The listing builds one solid part. Answer for the finished solid, in the listing's coordinates (mm). Face numbers are marked on the shaded views. A direction names the side the tool comes from. Round coordinates to 2 decimals unless told otherwise and drop trailing zeros. Loops run counter-clockwise (first coordinate to the right, second up) from the corner with the lowest first, then second, coordinate; pieces in that order, holes last. Notation, with made-up numbers: (33.25, 70) - (59.25, 70) arc R24 cw to (59.25, 91) - close; hole circle Ø10 at (-17, -9.5). An arc over 180 degrees is marked (long way). Write item = value, one per line. Start each with the question number.
1) Section C-C, the plane z = -34 is taken. Determine the outline of the cut face in (x, y).
2) Section D-D, the plane x = 6.25 is taken. Determine the outline of the cut face in (y, z), and give its area (3 significant figures).
3) Straight lines are drawn through the part: line 1 along Z through (x, y) = (12, 5.25); line 2 along Y through (x, z) = (-3, -8); line 3 along Z through (x, y) = (-7, -5). For each, find the intervals that lie inside material, in ascending order.
4) Given pin 1 Ø1.5 at (x, y) = (0.5, -7) entering from -Z; pin 2 Ø12 at (x, z) = (8.5, -1.5) entering from +Y; pin 3 Ø1.5 at (x, z) = (6.5, -31.5) entering from -Y; pin 4 Ø2 at (x, y) = (-7, 1) entering from +Z, each flat-ended and moving along its own axis, determine where each tip first touches the part or whether it passes through.
5) For a pull along X with two mould halves and no side action, classify the marked faces 4, 5, 6 and 7 as released by +X, released by -X, zero draft, split by the parting line, or undercut.
6) Section A-A, the plane z = -65 is taken. Determine the outline of the cut face in (x, y), and give its area (3 significant figures).
7) A tool of negligible diameter and unlimited length cuts with its end or side. For the marked faces 1, 2 and 3, from which of +Z, -Z, +X, -X, +Y, -Y can it reach the whole face along a straight path? Write none if from no direction.
8) Section B-B, the plane y = 0 is taken. Determine the outline of the cut face in (x, z), and give its area (3 significant figures).
from build123d import *

# Parameters (mm, degrees)
SKETCH_1_W          = 29.8
SKETCH_1_H          = 29.8
EXTRUDE_1_DEPTH     = 10
FILLET_1_R          = 10
SKETCH_2_W          = 10
SKETCH_2_H          = 10
EXTRUDE_2_DEPTH     = 70
SKETCH_3_W          = 5
SKETCH_3_H          = 10
CUT_EXTRUDE_1_DEPTH = 75.283376337
SKETCH_4_R          = 1.6
CUT_EXTRUDE_2_DEPTH = 75.283376337
CUT_EXTRUDE_3_DEPTH = 5
FILLET_3_R          = 2


with BuildPart() as part:
    # ｽｹｯﾁ1 → ﾎﾞｽ - 押し出し1 (new body)
    with BuildSketch(Plane.XY):
        Rectangle(SKETCH_1_W, SKETCH_1_H)
    extrude(amount=EXTRUDE_1_DEPTH)

    # ﾌｨﾚｯﾄ1
    fillet_1_edges = [part.edges().sort_by_distance(p)[0] for p in [
        (-14.9, -14.9, 5),
        (14.9, -14.9, 5),
        (14.9, 14.9, 5),
        (-14.9, 14.9, 5),
    ]]
    fillet(fillet_1_edges, radius=FILLET_1_R)

    # ｽｹｯﾁ2 → ﾎﾞｽ - 押し出し2 (add)
    with BuildSketch(Plane(origin=(0, 0, 0), x_dir=(-1, 0, 0), z_dir=(0, 0, -1))):
        Rectangle(SKETCH_2_W, SKETCH_2_H)
    extrude(amount=EXTRUDE_2_DEPTH)

    # ｽｹｯﾁ3 → ｶｯﾄ - 押し出し1 (cut, through all)
    with BuildSketch(Plane(origin=(0, 5, 0), x_dir=(1, 0, 0), z_dir=(0, 1, 0))):
        with Locations((0, 65)):
            Rectangle(SKETCH_3_W, SKETCH_3_H)
    extrude(amount=-CUT_EXTRUDE_1_DEPTH, mode=Mode.SUBTRACT)

    # ｽｹｯﾁ4 → ｶｯﾄ - 押し出し2 (cut, through all)
    with BuildSketch(Plane(origin=(5, 0, 0), x_dir=(0, 0, -1), z_dir=(1, 0, 0))):
        with Locations((65, 0)):
            Circle(SKETCH_4_R)
    extrude(amount=-CUT_EXTRUDE_2_DEPTH, mode=Mode.SUBTRACT)

    # ｽｹｯﾁ5 → ｶｯﾄ - 押し出し3 (cut)
    with BuildSketch(Plane.XY.offset(10)):
        with BuildLine():
            Line((-9.1, -10.1), (9.1, -10.1))
            ThreePointArc((9.1, -10.1), (9.807106781, -9.807106781), (10.1, -9.1))
            Line((10.1, -9.1), (10.1, 9.1))
            ThreePointArc((10.1, 9.1), (9.807106781, 9.807106781), (9.1, 10.1))
            Line((9.1, 10.1), (-9.1, 10.1))
            ThreePointArc((-9.1, 10.1), (-9.807106781, 9.807106781), (-10.1, 9.1))
            Line((-10.1, 9.1), (-10.1, -9.1))
            ThreePointArc((-10.1, -9.1), (-9.807106781, -9.807106781), (-9.1, -10.1))
        make_face()
    extrude(amount=-CUT_EXTRUDE_3_DEPTH, mode=Mode.SUBTRACT)

    # ﾌｨﾚｯﾄ3
    fillet_3_edges = [part.edges().sort_by_distance(p)[0] for p in [
        (-5, -5, -35),
        (-5, 5, -35),
        (5, 5, -35),
        (5, -5, -35),
    ]]
    fillet(fillet_3_edges, radius=FILLET_3_R)


solid = part.part
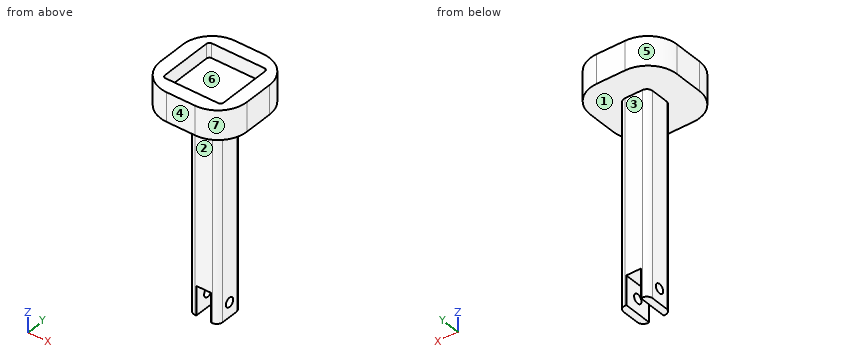
Geometry check:
q1.outline = (-5, -3) arc R2 ccw to (-3, -5) - (3, -5) arc R2 ccw to (5, -3) - (5, 3) arc R2 ccw to (3, 5) - (-3, 5) arc R2 ccw to (-5, 3) - close
q2.outline = (-14.81, 0) - (14.81, 0) - (14.81, 10) - (10.1, 10) - (10.1, 5) - (-10.1, 5) - (-10.1, 10) - (-14.81, 10) - close
q2.area = 195 mm2
q3.line_1 = 0 to 10
q3.line_2 = -5 to 5
q3.line_3 = 0 to 5
q4.pin_1 = 0
q4.pin_2 = 14.9
q4.pin_3 = through
q4.pin_4 = 5
q5.face_4 = zero draft
q5.face_5 = released by -X
q5.face_6 = undercut
q5.face_7 = released by +X
q6.outline = (-5, -3) arc R2 ccw to (-3, -5) - (-2.5, -5) - (-2.5, -1.6) - (-5, -1.6) - close; (-5, 1.6) - (-2.5, 1.6) - (-2.5, 5) - (-3, 5) arc R2 ccw to (-5, 3) - close; (2.5, -5) - (3, -5) arc R2 ccw to (5, -3) - (5, -1.6) - (2.5, -1.6) - close; (2.5, 1.6) - (5, 1.6) - (5, 3) arc R2 ccw to (3, 5) - (2.5, 5) - close
q6.area = 30.6 mm2
q7.face_1 = -Z
q7.face_2 = -Z, +X, -X, -Y
q7.face_3 = -Z, +X, -X, +Y
q8.outline = (-14.9, 0) - (-5, 0) - (-5, -63.4) - (-2.5, -63.4) - (-2.5, -60) - (2.5, -60) - (2.5, -63.4) - (5, -63.4) - (5, 0) - (14.9, 0) - (14.9, 10) - (10.1, 10) - (10.1, 5) - (-10.1, 5) - (-10.1, 10) - (-14.9, 10) - close; (-5, -70) - (-2.5, -70) - (-2.5, -66.6) - (-5, -66.6) - close; (2.5, -70) - (5, -70) - (5, -66.6) - (2.5, -66.6) - close
q8.area = 831 mm2
